Autodesk Inventor part; units mm, degrees
ref_plane "YZ Plane" through (0, 0, 0) normal (1, 0, 0) x (0, 1, 0)
ref_plane "XZ Plane" through (0, 0, 0) normal (0, 1, 0) x (-1, 0, 0)
ref_plane "XY Plane" through (0, 0, 0) normal (0, 0, 1) x (1, 0, 0)
sketch "Boceto1" plane through (0, 0, 0) normal (0, 1, 0) x (-1, 0, 0)
  line L0 (8.5, 0) -> (21, 0) construction
  line L1 (21, -7) -> (2.0913, -7)
  line L2 (21, -7) -> (27, -7)
  line L3 (21, 7) -> (27, 7)
  line L4 (27, 7) -> (27, -7)
  line L5 (27, -7) -> (32, -7)
  line L6 (32, -7) -> (32, 7)
  line L7 (32, 7) -> (27, 7)
  circle A0 centre (29.5, 0) radius 1
  line L8 (2.0913, -7) -> (2.0913, 7)
  line L9 (2.0913, -7) -> (16.0913, -7) construction
  line L10 (2.0913, 7) -> (21.0913, 7)
  line L11 (2.0913, -7) -> (-2.9087, -7)
  line L12 (2.0913, -7) -> (7.0913, -7) construction
  line L13 (-2.9087, -7) -> (-2.9087, 7)
  line L14 (-2.9087, 7) -> (2.0913, 7)
  circle A1 centre (-0.4087, 0) radius 1
  line L15 (2.0913, -7) -> (2.0913, 7)
  point P0 (0, 0)
  point P1 (0, 0)
  point P2 (0, 0)
  point P3 (0, 0)
  dimension "d3" = 6
  dimension "d5" = 5
  dimension "d6" = 14
  dimension "d7" = 2
  dimension "d8" = 14
  dimension "d9" = 90
  dimension "d10" = 19
  dimension "d11" = 5
  dimension "d12" = 180
  dimension "d13" = 14
  dimension "d14" = 2
extrude "Extrusión1" add sketch "Boceto1" along normal blind 18 contours L11 L13 L14 L8 | L4 L7 L6 L5
sketch "Boceto2" plane through (0, 0, 0) normal (0, -1, 0) x (1, 0, 0)
  line L0 (2.9087, 10) -> (-32, 10)
  line L1 (-32, 10) -> (-35, 10)
  line L2 (-35, 10) -> (-35, -7)
  line L3 (-35, -7) -> (-35, -10)
  line L4 (-35, -10) -> (2.9087, -10)
  line L5 (2.9087, -10) -> (5.9087, -10)
  line L6 (5.9087, -10) -> (5.9087, 10)
  line L7 (5.9087, 10) -> (2.9087, 10)
  line L8 (-2.0913, -7) -> (-27, -7)
  line L9 (-27, 7) -> (-2.0913, 7)
  line L10 (-2.0913, 7) -> (2.9087, 7)
  line L11 (2.9087, 7) -> (2.9087, -7)
  line L12 (2.9087, 7) -> (2.9087, -7)
  line L13 (2.9087, -7) -> (-2.0913, -7)
  line L14 (2.9087, -7) -> (-2.0913, -7)
  line L15 (-32, 7) -> (-27, 7)
  line L16 (-27, 7) -> (-32, 7)
  line L17 (-32, -7) -> (-32, 7)
  line L18 (-32, 7) -> (-32, -7)
  line L19 (-27, -7) -> (-32, -7)
  line L20 (-32, -7) -> (-27, -7)
  point P0 (0, 0)
  dimension "d21" = 3
  dimension "d22" = 3
  dimension "d23" = 3
extrude "Extrusión2" add sketch "Boceto2" against normal blind 23
sketch "Boceto3" plane through (0, 0, 0) normal (0, -1, 0) x (1, 0, 0)
  line L0 (5.9087, 10) -> (-35, 10)
  line L1 (5.9087, 10) -> (-35, 10)
  line L2 (-35, 10) -> (-35, -10)
  line L3 (-35, 10) -> (-35, -10)
  line L4 (-35, -10) -> (5.9087, -10)
  line L5 (5.9087, -10) -> (5.9087, 10)
  line L6 (5.9087, -10) -> (5.9087, 10)
  point P0 (0, 0)
extrude "Extrusión3" add sketch "Boceto3" along normal blind 3
sketch "Boceto4" plane through (0, 23, 0) normal (0, 1, 0) x (1, 0, 0)
  circle A0 centre (0.4087, 0) radius 1
  point P0 (0, 0)
extrude "Extrusión4" add sketch "Boceto4" along normal blind 15
sketch "Boceto5" plane through (0.4087, 38, 0) normal (0, 1, 0) x (1, 0, 0)
  circle A0 centre (-0.4087, 0) radius 10
  circle A1 centre (-0.4087, 0) radius 17.5
  line L0 (-35.4087, 10) -> (5.5, 10)
  line L1 (-35.4087, 10) -> (-35.4087, -10)
  line L2 (-35.4087, 10) -> (-35.4087, 14)
  line L3 (-35.4087, 14) -> (-10.9087, 14)
  line L4 (-10.9087, 14) -> (-5.5098, 8.6011)
  line L5 (-10.9087, 14) -> (-3.2735, 14) construction
  line L6 (5.5, -10) -> (-35.4087, -10)
  line L7 (-35.4087, -10) -> (-35.4087, -14)
  line L8 (-35.4087, -14) -> (-10.9087, -14)
  line L9 (-10.9087, -14) -> (-5.5098, -8.6011)
  line L10 (-10.9087, -14) -> (-3.2735, -14) construction
  dimension "d32" = 20
  dimension "d33" = 35
  dimension "d35" = 4
  dimension "d36" = 45
  dimension "d37" = 4
  dimension "d38" = 45
extrude "Extrusión5" add sketch "Boceto5" against normal blind 15 contours L4 L0 A0 | A0 L6 L9 | L0 L4 A1 L9 L6 A0 picked at (-3.4554, 12.4332)
sketch "Boceto6" plane through (0.4087, 38, 0) normal (0, 1, 0) x (1, 0, 0)
  circle A0 centre (0, 0) radius 1
  circle A1 centre (0, 0) radius 1
  point P0 (-0.4087, 0)
extrude "Extrusión6" cut sketch "Boceto6" against normal blind 15
sketch "Boceto7" plane through (0.4087, 23, 0) normal (0, -1, 0) x (1, 0, 0)
  circle A0 centre (-0.4087, 0) radius 17.5
  circle A1 centre (-0.4087, 0) radius 10
  line L0 (5.5, 8.0677) -> (5.5, -8.0677)
  arc A2 (-0.4087, -10) -> (5.5, -8.0677) centre (-0.4087, 0) ccw
  line L1 (5.5, 8.0677) -> (5.5, 10)
  line L2 (-35.4087, 10) -> (-6.9087, 10)
  line L3 (5.5, 10) -> (-6.9087, 10)
  line L4 (5.5, -8.0677) -> (5.5, -10)
  line L5 (5.5, -8.0677) -> (5.5, -10)
  line L6 (-0.4087, -10) -> (-6.9087, -10)
  line L7 (5.5, -10) -> (-6.9087, -10)
  arc A3 (-10.9087, -14) -> (-10.9087, 14) centre (-0.4087, 0) ccw
  line L8 (-10.9087, 14) -> (-10.9087, 10)
  line L9 (5.5, 10) -> (-35.4087, 10)
  line L10 (-10.9087, -14) -> (-10.9087, -10)
  line L11 (-10.9087, -10) -> (-6.9087, -10)
  line L12 (-6.9087, -10) -> (-35.4087, -10)
  dimension "d43" = 20
extrude "Extrusión7" add sketch "Boceto7" along normal blind 26 contours A0 L10 L11 L6 L7 L4 A1 L1 L3 L2 L8 | A1 L0 picked at (8.0064, 0)
sketch "Boceto8" plane through (0.4087, 38, 0) normal (0, 1, 0) x (1, 0, 0)
  line L0 (-0.4087, 0) -> (13.3413, 0)
  line L1 (-0.4087, 0) -> (8.4296, -10.5331)
  line L2 (-0.4087, 0) -> (13.3413, 0) construction
  line L3 (-0.4087, 0) -> (8.4296, 10.5331)
  line L4 (-0.4087, 0) -> (13.3413, 0) construction
  circle A0 centre (13.3413, 0) radius 1.75
  circle A1 centre (8.4296, -10.5331) radius 1.75
  circle A2 centre (8.4296, 10.5331) radius 1.75
  dimension "d46" = 13.75
  dimension "d47" = 13.75
  dimension "d48" = 50
  dimension "d49" = 13.75
  dimension "d50" = 50
  dimension "d51" = 3.5
  dimension "d52" = 3.5
  dimension "d53" = 3.5
extrude "Extrusión8" cut sketch "Boceto8" against normal blind 41
sketch "Boceto9" plane through (0, -3, 0) normal (0, -1, 0) x (1, 0, 0)
  circle A0 centre (8.8383, 10.5331) radius 1.75
  circle A1 centre (8.8383, 10.5331) radius 2.5
  circle A2 centre (13.75, 0) radius 1.75
  circle A3 centre (13.75, 0) radius 2.5
  circle A4 centre (8.8383, -10.5331) radius 1.75
  circle A5 centre (8.8383, -10.5331) radius 2.5
  point P0 (0, 0)
  dimension "d56" = 5
  dimension "d57" = 5
  dimension "d58" = 5
extrude "Extrusión9" cut sketch "Boceto9" against normal blind 36
properties part number "enganche_servo"
Model file for the job. Use its own axes, mm. A direction names the side the tool comes from. Give positions to 0.01 mm unless a question says otherwise; leave off trailing zeros. Loops run counter-clockwise (first coordinate to the right, second up) from the corner with the lowest first, then second, coordinate; pieces in that order, holes last. Notation, with made-up numbers: (84, -7) -> (106, -7) arc R6 cw to (106, -2) -> close; hole circle Ø3 at (9.25, 80.25). An arc over 180 degrees is marked (long way). Write each question's results on one line, items separated by ' | '.
(1) Tool access for faces 1 (the flat face through (12, 33, -1)), 2 (the flat face through (-23, 10, 10)), 3 (the flat face through (2.909, 20, 0)), 4 (the flat face through (-7.8, 30.6, -11.3)): list every direction of +Z, -Z, +X, -X, +Y, -Y with a clear straight run to the whole face (end or side of a thin tool).
Geometry results:
face 1: -Y | face 2: +Z, -X, +Y, -Y | face 3: +Y | face 4: -X, +Y
(2) Pull direction Z, two halves, no side cores. Call faces 5 (the cylindrical face through (-30.424, 8.874, 0.383)), 6 (the flat face through (-10.5, 10, -12)), 7 (the flat face through (-23, 10, -10)): released by +Z, released by -Z, zero draft, split by the parting line, or undercut.
Geometry results:
face 5: undercut | face 6: zero draft | face 7: released by -Z
(3) Flat gauge pins, fed straight in: pin 1 Ø14 at (x, z) = (-18, -3.5) entering from +Y; pin 2 Ø4 at (y, z) = (10.5, -3.5) entering from +X; pin 3 Ø1.8 at (x, z) = (-29.5, 0) entering from +Y; pin 4 Ø8 at (x, z) = (8.5, -12) entering from +Y. Where does each tip first touch, or does it go through?
Geometry results:
pin 1: stops at y = 23 | pin 2: stops at x = 17.44 | pin 3: stops at y = 0 | pin 4: stops at y = 38
(4) Cut at B-B on x = 13.75. List the corners of the cut face in (y, z), and give its area (3 significant figures).
Geometry results:
outline: (-3, -10.83) -> (38, -10.83) -> (38, -1.75) -> (33, -1.75) -> (33, -2.5) -> (-3, -2.5) -> close; (-3, 2.5) -> (33, 2.5) -> (33, 1.75) -> (38, 1.75) -> (38, 10.83) -> (-3, 10.83) -> close | area: 690 mm²
(5) Probe line 1 along Z through (x, y) = (9, 19.5); line 2 along Y through (x, z) = (-10, -6.5); line 3 along X through (y, z) = (34, -11.5). List the from-to ranges inside material, lowest first.
Geometry results:
line 1: z = -15.01 to -13.03, -8.04 to 8.04, 13.03 to 15.01 | line 2: y = -3 to 0 | line 3: x = -8 to 7.38, 10.3 to 13.19
(6) Cut at D-D on y = 8.5. List the corners of the cut face in (x, z), and give its area (3 significant figures).
Geometry results:
outline: (-35, -10) -> (-10.5, -10) -> (-10.5, -14) arc R17.5 ccw (long way) to (-10.5, 14) -> (-10.5, 10) -> (-35, 10) -> close; hole circle Ø2 at (-29.5, 0); hole (-27, -7) -> (-2.09, -7) -> (-2.09, 7) -> (-27, 7) -> close; hole circle Ø2 at (0.41, 0); hole circle Ø5 at (8.84, -10.53); hole circle Ø5 at (8.84, 10.53); hole circle Ø5 at (13.75, 0) | area: 901 mm²
(7) Cut at C-C on y = 35.5. List the corners of the cut face in (x, z).
Geometry results:
outline: (-10.5, -14) arc R17.5 ccw (long way) to (-10.5, 14) -> (-5.1, 8.6) arc R10 cw (long way) to (-5.1, -8.6) -> close; hole circle Ø3.5 at (8.84, -10.53); hole circle Ø3.5 at (8.84, 10.53); hole circle Ø3.5 at (13.75, 0)
